from build123d import *

# Parameters (mm, degrees)
F0_W     = 59.436
F0_H     = 124.46
F1_DEPTH = 7.62
F2_R     = 5.08
F4_DEPTH = 7.366


with BuildPart() as f1:
    # F0 (on Top) → F1 (new body)
    with BuildSketch(Plane.XY):
        with Locations((1.65762, 6.994029)):
            Rectangle(F0_W, F0_H)
    extrude(amount=F1_DEPTH)

    # F2
    f2_edges = [f1.edges().sort_by_distance(p)[0] for p in [
        (31.37562, -55.235971, 3.81),
        (-28.06038, -55.235971, 3.81),
        (31.37562, 69.224029, 3.81),
        (-28.06038, 69.224029, 3.81),
    ]]
    fillet(f2_edges, radius=F2_R)

    # F3 (on face) → F4 (join)
    with BuildSketch(Plane.XY.offset(7.62)):
        with BuildLine():
            Line((33.951722, 69.768132), (-24.722278, 69.768132))
            Line((-24.722278, 69.768132), (-24.722278, 68.916051))
            ThreePointArc((-24.722278, 68.916051), (-23.864837, 69.146442), (-22.98038, 69.224029))
            Line((-22.98038, 69.224029), (26.29562, 69.224029))
            ThreePointArc((26.29562, 69.224029), (29.887722, 67.736132), (31.37562, 64.144029))
            Line((31.37562, 64.144029), (31.37562, -50.155971))
            ThreePointArc((31.37562, -50.155971), (30.936819, -52.221321), (29.696222, -53.929868))
            Line((29.696222, -53.929868), (33.951722, -53.929868))
            Line((33.951722, -53.929868), (33.951722, 69.768132))
        make_face()
    extrude(amount=-F4_DEPTH)


solid = f1.part
For this review, take the finished solid that the model builds, in its own axes (mm). A direction names the side the tool comes from. Round coordinates to 2 decimals unless told otherwise and drop trailing zeros. Use a Markdown table: item, result. Add a question column.
Item 1: Tool access review of faces 1 (the flat face through (1, 8, 0)), 2 (the flat face through (32, -53.93, 4)): name each direction out of +Z, -Z, +X, -X, +Y, -Y from which nothing blocks a thin tool from reaching the whole face with its end or side.
Item 2: To check wall thickness, follow line 1 along Y through (x, z) = (26.5, 4.75); line 2 along X through (y, z) = (64.5, 3); line 3 along Y through (x, z) = (-24, 6.75). State the ranges of each line that lie inside material, in increasing order.
Item 3: Insertion check: pin 1 (0.7 mm diameter, centred on y = 69.5, z = 5.5, fed in from -X); pin 2 (4.5 mm diameter, centred on x = 31.5, z = 4, fed in from -Y). Each pin has a flat end and moves straight along its axis. Give the tip position at first contact, or say it passes through.
Geometry results:
| question | item | result |
|---|---|---|
| 1 | face 1 | -Z, +X, -X, +Y, -Y |
| 1 | face 2 | +Z, -Z, +X, -Y |
| 2 | line 1 | y = -55.23 to 69.77 |
| 2 | line 2 | x = -28.05 to 33.95 |
| 2 | line 3 | y = -55.13 to 69.77 |
| 3 | pin 1 | stops at x = -24.72 |
| 3 | pin 2 | stops at y = -54.29 |
